Model file for the job. Use its own axes, mm. Face numbers are marked on the shaded views. A direction names the side the tool comes from. Round coordinates to 2 decimals unless told otherwise and drop trailing zeros. Order: outer loops, then holes, each group sorted by start corner. A loop starts at its lowest first (then second) coordinate and runs counter-clockwise, first axis right, second up. Notation, with made-up numbers: (24.5, -5) -> (42.5, -5) arc R34 ccw to (42.5, 30) -> close; hole circle Ø10 at (84.5, 63.5). An arc over 180 degrees is marked (long way). Answer as CSV lines item,"result".
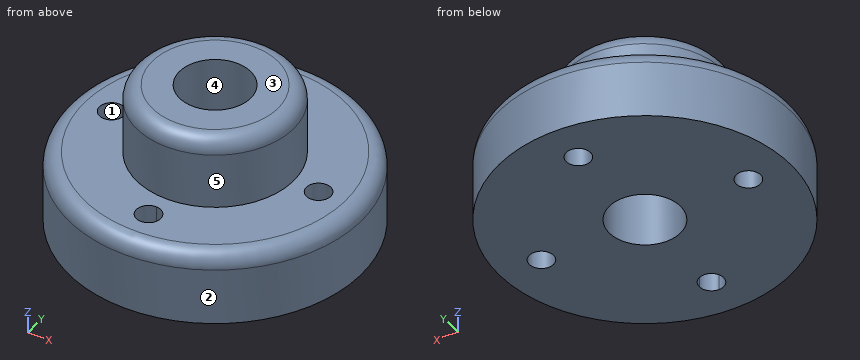
```python
from build123d import *

# Parameters (mm, degrees)
F0_R     = 30
F0_R_2   = 16.1
F1_DEPTH = 14.9
F2_DEPTH = 29.5
F3_R     = 3.2
F4_R     = 3.2
F5_R     = 2.5
F6_DEPTH = 100
F7_R     = 7.315
F8_DEPTH = 100


with BuildPart() as f1:
    # F0 (on Top) → F1 (new body)
    with BuildSketch(Plane.XY):
        Circle(F0_R)
        Circle(F0_R_2, mode=Mode.SUBTRACT)
    extrude(amount=F1_DEPTH)

    # F0 (on Top) → F2 (join)
    with BuildSketch(Plane.XY):
        Circle(F0_R_2)
    extrude(amount=F2_DEPTH)

    # F3
    f3_edges = [f1.edges().sort_by_distance(p)[0] for p in [
        (-30, 0, 14.9),
    ]]
    fillet(f3_edges, radius=F3_R)

    # F4
    f4_edges = [f1.edges().sort_by_distance(p)[0] for p in [
        (-16.1, 0, 29.5),
    ]]
    fillet(f4_edges, radius=F4_R)

    # F5 (on face) → F6 (cut)
    with BuildSketch(Plane.XY.offset(14.9)):
        with Locations((0, 21.45)):
            Circle(F5_R)
        with BuildLine():
            ThreePointArc((23.95, 0), (21.45, 2.5), (18.95, 0))
            ThreePointArc((18.95, 0), (21.45, -2.5), (23.95, 0))
        make_face()
        with BuildLine():
            ThreePointArc((2.5, -21.45), (1.767766953, -19.682233047), (0, -18.95))
            ThreePointArc((0, -18.95), (-2.5, -21.45), (0, -23.95))
            ThreePointArc((0, -23.95), (1.767766953, -23.217766953), (2.5, -21.45))
        make_face()
        with Locations((-21.45, 0)):
            Circle(F5_R)
    extrude(amount=-F6_DEPTH, mode=Mode.SUBTRACT)

    # F7 (on face) → F8 (cut)
    with BuildSketch(Plane.XY.offset(29.5)):
        Circle(F7_R)
    extrude(amount=-F8_DEPTH, mode=Mode.SUBTRACT)


solid = f1.part
```
Q1. Saw through at B-B (z = 23.75). Write the cut outline in (x, y) (3 decimals).
Checks:
outline,"circle Ø32.2 at (0, 0); hole circle Ø14.63 at (0, 0)"
Q2. Wall check: L1, parallel to Y at x = 0, z = 11.25 (3 decimals); L2, parallel to Z at x = -3, y = -23.5; L3, parallel to Y at x = 23, z = 6. Give the ranges that are in metal, low to high. Write a range as [from, to].
Checks:
L1,"[-30, -23.95], [-18.95, -7.315], [7.315, 18.95], [23.95, 30]"
L2,"[0, 14.9]"
L3,"[-19.26, -1.96], [1.96, 19.26]"
Q3. Tool access for the marked faces 4 and 5: list every direction of +Z, -Z, +X, -X, +Y, -Y with a clear straight run to the whole face (end or side of a thin tool).
Checks:
face 4,"+Z, -Z"
face 5,"+Z"
Q4. Saw through at C-C (z = 13). Write the cut outline in (x, y) (3 decimals), plus the area to 3 significant figures.
Checks:
outline,"circle Ø59.448 at (0, 0); hole circle Ø5 at (-21.45, 0); hole circle Ø14.63 at (0, 0); hole circle Ø5 at (0, -21.45); hole circle Ø5 at (0, 21.45); hole circle Ø5 at (21.45, 0)"
area,"2,530 mm²"
Q5. Saw through at A-A (z = 3). Write the cut outline in (x, y) (3 decimals), plus the area to 3 significant figures.
Checks:
outline,"circle Ø60 at (0, 0); hole circle Ø5 at (-21.45, 0); hole circle Ø14.63 at (0, 0); hole circle Ø5 at (0, -21.45); hole circle Ø5 at (0, 21.45); hole circle Ø5 at (21.45, 0)"
area,"2,580 mm²"
Q6. Mould opens along X. For the marked faces 1, 2 and 3 say: +X half, -X half, draft (parallel to the pull), parting line (faces both ways), or undercut.
Checks:
face 1,"undercut"
face 2,"parting line"
face 3,"draft"
Q7. Flat gauge pins, fed straight in: pin 1 (10 mm diameter, centred on y = -14, z = 3.5, fed in from +X); pin 2 (6.5 mm diameter, centred on x = 0, y = 21.45, fed in from -Z); pin 3 (10 mm diameter, centred on y = -0.5, z = 17, fed in from -X); pin 4 (10 mm diameter, centred on x = 18, z = 24.5, fed in from -Y). Where does each tip first touch, or does it go through?
Checks:
pin 1,"x = 28.62"
pin 2,"z = 0"
pin 3,"x = -29.98"
pin 4,"y = -9.5"
